from build123d import *

# Parameters (mm, degrees)
BOSS_EXTRUDE1_DEPTH = 50
BOSS_EXTRUDE2_DEPTH = 50


with BuildPart() as part:
    # Sketch1 → Boss-Extrude1 (new body)
    with BuildSketch(Plane.XY):
        Polygon((0, 0), (2, 0), (2, 2), (8, 12), (-6, 12), (0, 2), align=None)
    extrude(amount=BOSS_EXTRUDE1_DEPTH)

    # Sketch2 → Boss-Extrude2 (add)
    with BuildSketch(Plane.XY.offset(50)):
        with BuildLine():
            Line((-6, 12), (8, 12))
            ThreePointArc((8, 12), (1, 14.858571571), (-6, 12))
        make_face()
    extrude(amount=-BOSS_EXTRUDE2_DEPTH)


solid = part.part
Input: part model. Units: mm. Frame: model coordinates. A direction names the side the tool comes from. Give positions to 0.01 mm unless a question says otherwise; leave off trailing zeros. Write each loop counter-clockwise with the first axis right and the second up, starting at its lowest first coordinate (ties: lowest second). Pieces come first, ordered by that corner, then holes.
Q1. First-contact query: P1, Ø1, axis at y = 0.5, z = 22.5, coming from the -X side; P2, Ø3, axis at x = -4, z = 41.5, coming from the +Y side; P3, Ø2, axis at x = 6, z = 16.5, coming from the +Y side. Flat tips, straight axial feed; report the tip coordinate or a pass-through.
Q2. Material intervals for probe 1 along Y at (x, z) = (1.25, 37.5); probe 2 along X at (y, z) = (3.5, 38.5); probe 3 along X at (y, z) = (7.5, 23), sorted ascending.
Q3. Section C-C, the plane x = -4.25. Output: boundary loops of the cut face in (y, z).
Q4. Section A-A, the plane z = 25.5. Output: boundary loops of the cut face in (x, y).
Q5. Section B-B, the plane y = 5. Output: boundary loops of the cut face in (x, z).
Q6. Set-up query: faces 4 (the face through (0, 1, 25)), 5 (the face through (1, 0, 25)), 6 (the face through (2, 1, 25)). Return all of +Z, -Z, +X, -X, +Y, -Y with unobstructed straight access to the full face (end or side cutting, diameter ignored); none if empty.
Q7. Pull-direction query (Y, two-part tool) for faces 1 (the face through (-3, 7, 25)), 2 (the face through (1.109, 14.858, 25.35)), 3 (the face through (1, 9, 0)); classes: pulls with the +Y half, pulls with the -Y half, needs draft (parallel to the pull), parting line crosses it, or undercut.
Filled in:
1. P1: stops at x = 0
1. P2: stops at y = 14.23
1. P3: stops at y = 14.02
2. probe 1: y = 0 to 14.86
2. probe 2: x = -0.9 to 2.9
2. probe 3: x = -3.3 to 5.3
3. outline: (9.08, 0) - (13.37, 0) - (13.37, 50) - (9.08, 50) - close
4. outline: (-6, 12) - (0, 2) - (0, 0) - (2, 0) - (2, 2) - (8, 12) arc R10 ccw to start
5. outline: (-1.8, 0) - (3.8, 0) - (3.8, 50) - (-1.8, 50) - close
6. face 4: +Z, -Z, -X, -Y
6. face 5: +Z, -Z, +X, -X, -Y
6. face 6: +Z, -Z, +X, -Y
7. face 1: pulls with the -Y half
7. face 2: pulls with the +Y half
7. face 3: needs draft
